Read the model definition and answer for the solid it produces. Units are mm, in the model's axes. A direction names the side the tool comes from. Give positions to 0.01 mm unless a question says otherwise; leave off trailing zeros. Write each loop counter-clockwise with the first axis right and the second up, starting at its lowest first coordinate (ties: lowest second). Pieces come first, ordered by that corner, then holes. Notation, with made-up numbers: (65.5, 13.5) -> (124.5, 13.5) arc R23 cw to (124.5, 23.5) -> close; hole circle Ø6 at (13, 41.5). An arc over 180 degrees is marked (long way). Use a Markdown table: item, result.
from build123d import *

# Parameters (mm, degrees)
CYLINDER_R        = 2.1
CYLINDER_DEPTH    = 100
CYLINDER006_R     = 5.5
CYLINDER006_DEPTH = 15
CYLINDER007_R     = 6.5
CYLINDER007_DEPTH = 2


with BuildPart() as centeraxis:
    # Cylinder → Cylinder (new body)
    with BuildSketch(Plane.XY.offset(-10)):
        Circle(CYLINDER_R)
    extrude(amount=CYLINDER_DEPTH)


with BuildPart() as bearing003:
    # Cylinder006 → Cylinder006 (new body)
    with BuildSketch(Plane.XY.offset(21)):
        Circle(CYLINDER006_R)
    extrude(amount=CYLINDER006_DEPTH)


with BuildPart() as centerbearing001:
    # Cylinder007 → Cylinder007 (new body)
    with BuildSketch(Plane.XY.offset(21)):
        Circle(CYLINDER007_R)
    extrude(amount=CYLINDER007_DEPTH)

    # Fusion001: union Bearing003
    add(bearing003.part)

    # Cut012: cut CenterAxis
    add(centeraxis.part, mode=Mode.SUBTRACT)


with BuildPart() as centerbearing001_1:
    # Cut012 placement: moved
    add(centerbearing001.part.moved(Location((-60, 0, 0))))


solid = centerbearing001_1.part
Item 1: A cutting plane is placed at A-A (x = -60). Give the vertices of the cut face in (y, z).
Return value:
| item | result |
|---|---|
| outline | (-6.5, 21) -> (-2.1, 21) -> (-2.1, 36) -> (-5.5, 36) -> (-5.5, 23) -> (-6.5, 23) -> close; (2.1, 21) -> (6.5, 21) -> (6.5, 23) -> (5.5, 23) -> (5.5, 36) -> (2.1, 36) -> close |
Item 2: Each of these flat-tipped pins is pushed along its axis until it touches: P1, Ø5, axis at x = -56.5, z = 26, coming from the -Y side; P2, Ø4, axis at y = -1.5, z = 25.5, coming from the +X side; P3, Ø5, axis at y = 1, z = 24, coming from the -X side; P4, Ø2, axis at x = -55.5, z = 31, coming from the -Y side. Where does it stop, or does it pass through?
Return value:
| item | result |
|---|---|
| P1 | y = -5.41 |
| P2 | x = -54.5 |
| P3 | x = -66.5 |
| P4 | y = -4.24 |
Item 3: A cutting plane is placed at B-B (y = 0). Give the vertices of the cut face in (x, z), then the cut area to 3 significant figures.
Return value:
| item | result |
|---|---|
| outline | (-66.5, 21) -> (-62.1, 21) -> (-62.1, 36) -> (-65.5, 36) -> (-65.5, 23) -> (-66.5, 23) -> close; (-57.9, 21) -> (-53.5, 21) -> (-53.5, 23) -> (-54.5, 23) -> (-54.5, 36) -> (-57.9, 36) -> close |
| area | 106 mm^2 |
Item 4: A cutting plane is placed at C-C (z = 34.5). Give the vertices of the cut face in (x, y), then the cut area to 3 significant figures.
Return value:
| item | result |
|---|---|
| outline | circle Ø11 at (-60, 0); hole circle Ø4.2 at (-60, 0) |
| area | 81.2 mm^2 |
Item 5: A tool of negligible diameter and unlimited length cuts with its end or side. For faces 4 (the face through (-62, 2, 21)), 5 (the face through (-65.495, 0.242, 29.409)), from which of +Z, -Z, +X, -X, +Y, -Y can it reach the whole face along a straight path? Write none if from no direction.
Return value:
| item | result |
|---|---|
| face 4 | -Z, +X, -X, +Y, -Y |
| face 5 | +Z |
Item 6: A cutting plane is placed at D-D (x = -63.75). Give the vertices of the cut face in (y, z), then the cut area to 3 significant figures.
Return value:
| item | result |
|---|---|
| outline | (-5.31, 21) -> (5.31, 21) -> (5.31, 23) -> (4.02, 23) -> (4.02, 36) -> (-4.02, 36) -> (-4.02, 23) -> (-5.31, 23) -> close |
| area | 126 mm^2 |
Item 7: Straight lines are drawn through the part: line 1 along X through (y, z) = (0, 27.5); line 2 along Y through (x, z) = (-60, 26.75); line 3 along Z through (x, y) = (-56.5, 4.5). For each, find the intervals that lie inside material, in ascending order. Write a range as [from, to].
Return value:
| item | result |
|---|---|
| line 1 | [-65.5, -62.1], [-57.9, -54.5] |
| line 2 | [-5.5, -2.1], [2.1, 5.5] |
| line 3 | [21, 23] |
Item 8: For a pull along Y with two mould halves and no side action, classify faces 1 (the face through (-53.8, 1.95, 21.99)), 2 (the face through (-58.06, -0.8, 28.39)), 3 (the face through (-57.6, 0.1, 36)) as +Y half, -Y half, draft (parallel to the pull), parting line (faces both ways), or undercut.
Return value:
| item | result |
|---|---|
| face 1 | parting line |
| face 2 | undercut |
| face 3 | draft |
